Read the model definition and answer for the solid it produces. Units are mm, in the model's axes. Face numbers are marked on the shaded views. A direction names the side the tool comes from. Coordinates: 2 decimals unless noted, no trailing zeros. Write each loop counter-clockwise with the first axis right and the second up, starting at its lowest first coordinate (ties: lowest second). Pieces come first, ordered by that corner, then holes. Notation, with made-up numbers: (-29, -24.5) -> (18, -24.5) arc R12 cw to (18, -12.5) -> close; hole circle Ø5 at (31.5, 18). An arc over 180 degrees is marked (long way). Answer as a JSON object with one key per item and string values. Group by question number.
(1) Find section D-D (z = 23.5). Give the vertices of the cut face in (x, y).
(2) Find section C-C (y = 85.5). Give the vertices of the cut face in (x, z), then the cut area to 3 significant figures.
(3) Find section A-A (x = -31.5). Give the vertices of the cut face in (y, z).
(4) Find section B-B (z = 17.5). Give the vertices of the cut face in (x, y).
(5) Which of the six approach directions +Z, -Z, +X, -X, +Y, -Y give full straight-line access (tool end or side, diameter ignored) to the marked faces 3, 4 and 5?
(6) For a pull along Y with two mould halves and no side action, classify the marked faces 1 and 2 as +Y half, -Y half, draft (parallel to the pull), parting line (faces both ways), or undercut.
(7) Straight lines are drawn through the part: L1, parallel to Z at x = -28, y = 92; L2, parallel to Y at x = -5, z = 26; L3, parallel to Z at x = 7.5, y = 85.5. For each, find the intervals that lie inside material, in ascending order.
(8) Flat-ended cylindrical pins translate along their axes: P1, Ø5, axis at x = -12.5, z = 14.5, coming from the +Y side; P2, Ø4.5, axis at x = 7.82, y = 93.63, coming from the +Z side; P3, Ø3, axis at y = 55, z = 2, coming from the +X side; P4, Ø1.5, axis at y = 6.5, z = 1, coming from the +X side. Find the tip coordinate at first contact, or state that the pin passes through.
from build123d import *

# Parameters (mm, degrees)
F0_R      = 1.75
F0_R_2    = 2
F1_DEPTH  = 4
F2_DEPTH  = 3
F0_R_3    = 1.6666666667
F3_DEPTH  = 1.9
F4_DEPTH  = 33
F5_R      = 2
F9_R      = 1.5
F10_DEPTH = 25
F8_R      = 1.5
F11_DEPTH = 25


with BuildPart() as f1:
    # F0 (on Top) → F1 (new body)
    with BuildSketch(Plane.XY):
        Polygon((26.8151908007, 97.6259698881), (-25.1848091993, 97.6259698881), (-50.1848091993, 97.6259698881), (-50.1848091993, 89.6259698881), (-25.1848091993, 89.6259698881), (-25.1848091993, 23.6259698881), (-50.1848091993, 23.6259698881), (-50.1848091993, 15.6259698881), (-25.1848091993, 15.6259698881), (-4.1848091993, 15.6259698881), (5.8151908007, 15.6259698881), (26.8151908007, 15.6259698881), (51.8151908007, 15.6259698881), (51.8151908007, 23.6259698881), (26.8151908007, 23.6259698881), (26.8151908007, 89.6259698881), (51.8151908007, 89.6259698881), (51.8151908007, 97.6259698881), align=None)
        with Locations((-37.6848091993, 19.6259698881)):
            Circle(F0_R, mode=Mode.SUBTRACT)
        with Locations((39.3151908007, 19.6259698881)):
            Circle(F0_R, mode=Mode.SUBTRACT)
        with Locations((-37.6848091993, 93.6259698881)):
            Circle(F0_R, mode=Mode.SUBTRACT)
        with Locations((-6.1848091993, 93.6259698881)):
            Circle(F0_R_2, mode=Mode.SUBTRACT)
        Polygon((10.2151908007, 67.7759698881), (24.3151908007, 67.7759698881), (24.3151908007, 25.4759698881), (-22.6848091993, 25.4759698881), (-22.6848091993, 42.9759698881), (10.2151908007, 42.9759698881), (10.2151908007, 58.7915498881), (5.2151908007, 58.7915498881), (5.2151908007, 68.7915498881), (10.2151908007, 68.7915498881), align=None, mode=Mode.SUBTRACT)
        Polygon((24.3151908007, 70.2759698881), (10.2151908007, 70.2759698881), (7.2151908007, 70.2759698881), (-8.5848091993, 70.2759698881), (-8.5848091993, 54.4603863134), (-3.5848091993, 54.4603863134), (-3.5848091993, 44.4603863134), (-8.5848091993, 44.4603863134), (-8.5848091993, 45.4759698881), (-22.6848091993, 45.4759698881), (-22.6848091993, 87.7759698881), (24.3151908007, 87.7759698881), align=None, mode=Mode.SUBTRACT)
        with Locations((7.8151908007, 93.6259698881)):
            Circle(F0_R_2, mode=Mode.SUBTRACT)
        with Locations((39.3151908007, 93.6259698881)):
            Circle(F0_R, mode=Mode.SUBTRACT)
    extrude(amount=F1_DEPTH)

    # F0 (on Top) → F2 (join)
    with BuildSketch(Plane.XY):
        Polygon((24.3151908007, 25.4759698881), (24.3151908007, 67.7759698881), (10.2151908007, 67.7759698881), (10.2151908007, 61.4111642682), (10.2151908007, 58.7915498881), (10.2151908007, 42.9759698881), (-22.6848091993, 42.9759698881), (-22.6848091993, 25.4759698881), align=None)
        Polygon((7.2151908007, 70.2759698881), (10.2151908007, 70.2759698881), (24.3151908007, 70.2759698881), (24.3151908007, 87.7759698881), (-22.6848091993, 87.7759698881), (-22.6848091993, 45.4759698881), (-8.5848091993, 45.4759698881), (-8.5848091993, 54.4603863134), (-8.5848091993, 70.2759698881), align=None)
    extrude(amount=F2_DEPTH)

    # F0 (on Top) → F3 (join)
    with BuildSketch(Plane.XY):
        with BuildLine():
            Line((5.8151908007, 15.6259698881), (-4.1848091993, 15.6259698881))
            Line((-4.1848091993, 15.6259698881), (-4.1848091993, -4.3740301119))
            ThreePointArc((-4.1848091993, -4.3740301119), (0.8151908007, -9.3740301119), (5.8151908007, -4.3740301119))
            Line((5.8151908007, -4.3740301119), (5.8151908007, 15.6259698881))
        make_face()
        with Locations((0.8151908007, -4.3740301119)):
            Circle(F0_R_3, mode=Mode.SUBTRACT)
    extrude(amount=F3_DEPTH)

    # F0 (on Top) → F4 (join)
    with BuildSketch(Plane.XY):
        Polygon((10.2151908007, 61.4111642682), (10.2151908007, 67.7759698881), (10.2151908007, 68.7915498881), (5.2151908007, 68.7915498881), (5.2151908007, 58.7915498881), (10.2151908007, 58.7915498881), align=None)
        Polygon((-3.5848091993, 54.4603863134), (-8.5848091993, 54.4603863134), (-8.5848091993, 45.4759698881), (-8.5848091993, 44.4603863134), (-3.5848091993, 44.4603863134), align=None)
    extrude(amount=F4_DEPTH)

    # F5
    f5_edges = [f1.edges().sort_by_distance(p)[0] for p in [
        (51.815191, 97.62597, 2),
        (-50.184809, 97.62597, 2),
        (-50.184809, 89.62597, 2),
        (-50.184809, 15.62597, 2),
        (51.815191, 23.62597, 2),
        (51.815191, 15.62597, 2),
        (51.815191, 89.62597, 2),
        (-50.184809, 23.62597, 2),
    ]]
    fillet(f5_edges, radius=F5_R)

    # F9 (on offset) → F10 (cut)
    with BuildSketch(Plane(origin=(-8.5848091993, 0, 0), x_dir=(0, -1, 0), z_dir=(-1, 0, 0))):
        with Locations((-49.4603863134, 23.5)):
            Circle(F9_R)
        with Locations((-49.4603863134, 5.5)):
            Circle(F9_R)
    extrude(amount=-F10_DEPTH, mode=Mode.SUBTRACT)

    # F8 (on offset) → F11 (cut)
    with BuildSketch(Plane.YZ.offset(10.2151908007)):
        with Locations((63.7915498881, 5.5)):
            Circle(F8_R)
        with Locations((63.7915498881, 23.5)):
            Circle(F8_R)
    extrude(amount=-F11_DEPTH, mode=Mode.SUBTRACT)


solid = f1.part
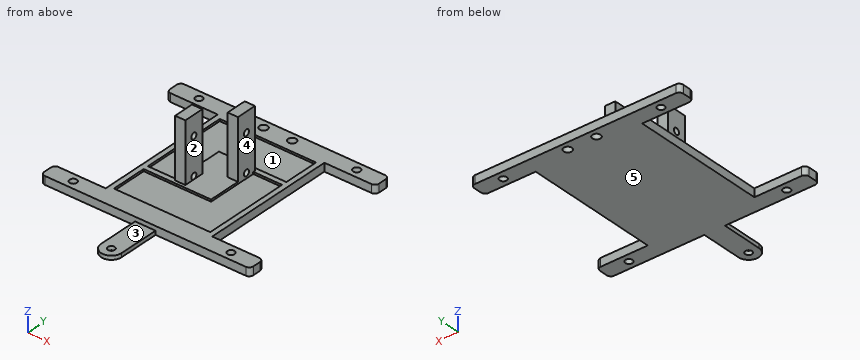
Results below:
{
 "1": {"outline": "(-8.58, 44.46) -> (-3.58, 44.46) -> (-3.58, 47.96) -> (-8.58, 47.96) -> close; (-8.58, 50.96) -> (-3.58, 50.96) -> (-3.58, 54.46) -> (-8.58, 54.46) -> close; (5.22, 58.79) -> (10.22, 58.79) -> (10.22, 62.29) -> (5.22, 62.29) -> close; (5.22, 65.29) -> (10.22, 65.29) -> (10.22, 68.79) -> (5.22, 68.79) -> close"},
 "2": {"outline": "(-25.18, 0) -> (26.82, 0) -> (26.82, 4) -> (24.32, 4) -> (24.32, 3) -> (-22.68, 3) -> (-22.68, 4) -> (-25.18, 4) -> close", "area": "161 mm2"},
 "3": {"outline": "(15.63, 0) -> (23.63, 0) -> (23.63, 4) -> (15.63, 4) -> close; (89.63, 0) -> (97.63, 0) -> (97.63, 4) -> (89.63, 4) -> close"},
 "4": {"outline": "(-8.58, 44.46) -> (-3.58, 44.46) -> (-3.58, 54.46) -> (-8.58, 54.46) -> close; (5.22, 58.79) -> (10.22, 58.79) -> (10.22, 68.79) -> (5.22, 68.79) -> close"},
 "5": {"face 3": "+Z, +X, -X, -Y", "face 4": "+Z", "face 5": "-Z, +X, -X, +Y, -Y"},
 "6": {"face 1": "undercut", "face 2": "draft"},
 "7": {"L1": "z = 0 to 4", "L2": "y = 44.46 to 54.46", "L3": "z = 0 to 3"},
 "8": {"P1": "passes through", "P2": "stops at z = 4", "P3": "stops at x = 26.82", "P4": "stops at x = 5.82"}
}
